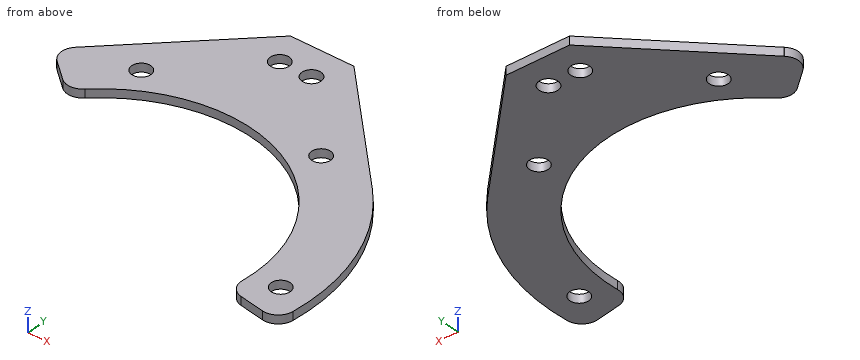
```python
from build123d import *

# Parameters (mm, degrees)
SKETCH1_R                = 39.5
BOSS_EXTRUDE1_DEPTH      = 0.79375
BOSS_EXTRUDE2_DEPTH      = 1.5875
SKETCH2_R                = 28.75
CUT_EXTRUDE1_DEPTH       = 64.739863165
M3_CLEARANCE_HOLE1_D     = 3.6
CIRPATTERN1_COUNT        = 6
M3_CLEARANCE_HOLE2_D     = 3.6
M3_CLEARANCE_HOLE2_DEPTH = 10
M3_CLEARANCE_HOLE2_TIP   = 1.081549114
CUT_EXTRUDE3_DEPTH       = 64.739863165
FILLET1_R                = 3


with BuildPart() as part:
    # Sketch1 → Boss-Extrude1 (new, symmetric)
    with BuildSketch(Plane.XY):
        Circle(SKETCH1_R)
    extrude(amount=BOSS_EXTRUDE1_DEPTH, both=True)

    # Sketch3 → Boss-Extrude2 (add, through all)
    with BuildSketch(Plane.XY.offset(0.79375)):
        Polygon((-28.01836343, 27.842796388), (-6, 50), (6, 50), (28.01836343, 27.842796388), align=None)
    extrude(amount=-BOSS_EXTRUDE2_DEPTH)

    # Sketch2 → Cut-Extrude1 (cut, through all)
    with BuildSketch(Plane.XY.offset(0.79375)):
        Circle(SKETCH2_R)
    extrude(amount=-CUT_EXTRUDE1_DEPTH, mode=Mode.SUBTRACT)

    # M3 Clearance Hole1 (through all)
    with Locations(Plane.XY.offset(0.79375)):
        with Locations((17, -29.444863729)):
            m3_clearance_hole1 = Hole(M3_CLEARANCE_HOLE1_D / 2)

    # CirPattern1: M3 Clearance Hole1 ×6 about axis
    cirpattern1_axis = Axis((0, 0, 0), (0, 0, 1))
    for i in range(1, CIRPATTERN1_COUNT):
        add(m3_clearance_hole1.rotate(cirpattern1_axis, i * 360 / CIRPATTERN1_COUNT), mode=Mode.SUBTRACT)

    # M3 Clearance Hole2
    with Locations(Plane.XY.offset(0.79375)):
        with Locations((3, 44), (-3, 44)):
            Hole(M3_CLEARANCE_HOLE2_D / 2, depth=M3_CLEARANCE_HOLE2_DEPTH)
            with Locations((0, 0, -(M3_CLEARANCE_HOLE2_DEPTH + M3_CLEARANCE_HOLE2_TIP / 2))):  # 118° drill point
                Cone(0, M3_CLEARANCE_HOLE2_D / 2, M3_CLEARANCE_HOLE2_TIP, mode=Mode.SUBTRACT)

    # OpenEdge → Cut-Extrude3 (cut, through all)
    with BuildSketch(Plane(origin=(0, 0, -0.79375), x_dir=(-1, 0, 0), z_dir=(0, 0, -1))):
        with BuildLine():
            Line((22.02377774, 18.480143778), (30.258755503, 25.390110583))
            ThreePointArc((30.258755503, 25.390110583), (16.693421339, -35.799157588), (-38.899906244, -6.859103018))
            Line((-38.899906244, -6.859103018), (-28.313222899, -4.992385108))
            ThreePointArc((-28.313222899, -4.992385108), (12.150275025, -26.056348877), (22.02377774, 18.480143778))
        make_face()
    extrude(amount=-CUT_EXTRUDE3_DEPTH, mode=Mode.SUBTRACT)

    # Fillet1
    fillet1_edges = [part.edges().sort_by_distance(p)[0] for p in [
        (28.313222899, -4.992385108, 0),
        (-22.02377774, 18.480143778, 0),
        (-30.258755503, 25.390110583, 0),
        (38.899906244, -6.859103018, 0),
    ]]
    fillet(fillet1_edges, radius=FILLET1_R)


solid = part.part
```
The listing builds one solid part. Answer for the finished solid, in the listing's coordinates (mm). Give positions to 0.01 mm unless a question says otherwise; leave off trailing zeros. Order: outer loops, then holes, each group sorted by start corner. A loop starts at its lowest first (then second) coordinate and runs counter-clockwise, first axis right, second up. Notation, with made-up numbers: (3, -7) -> (13, -7) arc R3 cw to (13, -2) -> close; hole circle Ø7 at (-37.75, -14). An arc over 180 degrees is marked (long way). Answer as a JSON object with one key per item and string values. Group by question number.
Item 1: Consider L1, parallel to Y at x = 34, z = -0.1; L2, parallel to Y at x = 4, z = 0.2; L3, parallel to X at y = 30, z = -0.6. Determine where each line is inside the solid, lowest interval first. Write a range as from..to.
Item 2: The part is cut by section A-A on y = 0. Write down the section's boundary in (x, z).
Item 3: The part is cut by section C-C on z = -0.5. Write down the section's boundary in (x, y).
Item 4: The part is cut by section B-B on x = 17. Write down the section's boundary in (y, z).
Item 5: A flat-ended cylindrical pin translates along its axis: pin 1 (3 mm diameter, centred on x = 17, y = 29.44, fed in from -Z). Find the tip coordinate at first contact, or state that the pin passes through.
Item 6: The part is cut by section D-D on y = 44. Write down the section's boundary in (x, z), and give its area (3 significant figures).
Result set:
{
 "1": {"L1": "-6..-1.8, 1.8..20.11", "L2": "28.47..42.5, 45.5..50", "L3": "-25.87..-18.71, -15.29..15.29, 18.71..25.87"},
 "2": {"outline": "(28.75, -0.79) -> (32.2, -0.79) -> (32.2, 0.79) -> (28.75, 0.79) -> close; (35.8, -0.79) -> (39.5, -0.79) -> (39.5, 0.79) -> (35.8, 0.79) -> close"},
 "3": {"outline": "(-28.07, 27.79) arc R3 ccw to (-27.87, 23.38) -> (-24.21, 20.32) arc R3 ccw to (-20.18, 20.48) arc R28.75 cw to (28.66, -2.29) arc R3 ccw to (31.13, -5.49) -> (35.82, -6.32) arc R3 ccw to (39.33, -3.64) arc R39.5 ccw to (28.02, 27.84) -> (6, 50) -> (-6, 50) -> (-28.02, 27.84) arc R39.5 ccw to start; hole circle Ø3.6 at (-17, 29.44); hole circle Ø3.6 at (-3, 44); hole circle Ø3.6 at (3, 44); hole circle Ø3.6 at (17, 29.44); hole circle Ø3.6 at (34, 0)"},
 "4": {"outline": "(23.19, -0.79) -> (27.64, -0.79) -> (27.64, 0.79) -> (23.19, 0.79) -> close; (31.24, -0.79) -> (38.93, -0.79) -> (38.93, 0.79) -> (31.24, 0.79) -> close"},
 "5": {"pin 1": "through"},
 "6": {"outline": "(-11.96, -0.79) -> (-4.8, -0.79) -> (-4.8, 0.79) -> (-11.96, 0.79) -> close; (-1.2, -0.79) -> (1.2, -0.79) -> (1.2, 0.79) -> (-1.2, 0.79) -> close; (4.8, -0.79) -> (11.96, -0.79) -> (11.96, 0.79) -> (4.8, 0.79) -> close", "area": "26.6 mm²"}
}
